Study the drawing (mm; zero at the part's minimum x, y, z) and answer. Coordinates: 2 decimals unless noted, no trailing zeros. Loops run counter-clockwise (first coordinate to the right, second up) from the corner with the lowest first, then second, coordinate; pieces in that order, holes last. Notation, with made-up numbers: (67.5, 84) - (100.5, 84) arc R15 ccw to (100.5, 105) - close; hole circle Ø1 at (77.25, 26). An arc over 180 degrees is marked (long way). Put each result on its own line as item: value.
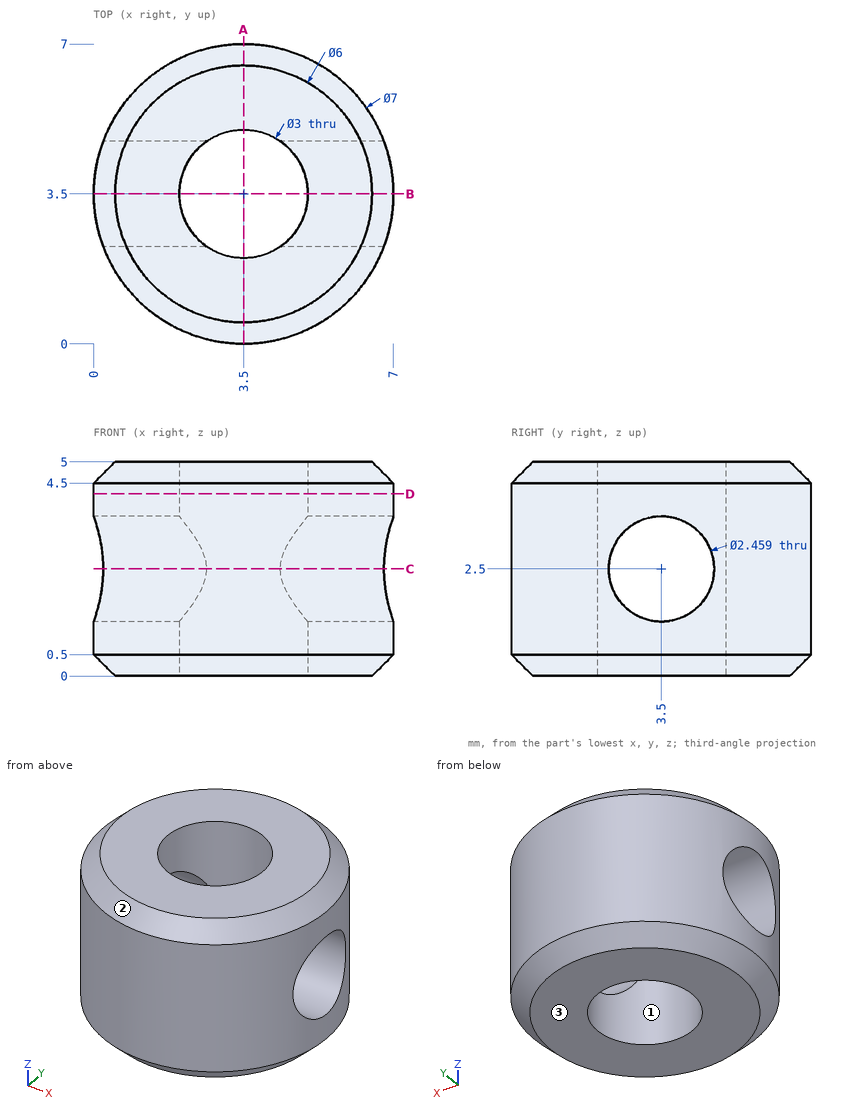
1) For a pull along Y with two mould halves and no side action, classify the marked faces 1, 2 and 3 as pulls with the +Y half, pulls with the -Y half, needs draft (parallel to the pull), parting line crosses it, or undercut.
Found:
face 1: undercut
face 2: parting line crosses it
face 3: needs draft
2) Straight lines are drawn through the part: L1, parallel to Y at x = 3, z = 1.5; L2, parallel to Y at x = 1.25, z = 2.5. For each, find the intervals that lie inside material, in ascending order. Write a range as [from, to].
Found:
L1: y = [0.04, 2.09], [4.91, 6.96]
L2: y = [0.82, 2.27], [4.73, 6.18]
3) The part is cut by section B-B (y = 3.5). Give the vertices of the cut face in (x, z).
Found:
outline: (0, 0.5) - (0.5, 0) - (2, 0) - (2, 1.27) - (0, 1.27) - close; (0, 3.73) - (2, 3.73) - (2, 5) - (0.5, 5) - (0, 4.5) - close; (5, 0) - (6.5, 0) - (7, 0.5) - (7, 1.27) - (5, 1.27) - close; (5, 3.73) - (7, 3.73) - (7, 4.5) - (6.5, 5) - (5, 5) - close
4) Each of these flat-tipped pins is pushed along its axis until it touches: pin 1 (1 mm diameter, centred on x = 6.5, y = 1.5, fed in from +Z); pin 2 (1.8 mm diameter, centred on x = 3.5, y = 3.5, fed in from +Z). Where does it stop, or does it pass through?
Found:
pin 1: stops at z = 4.89
pin 2: passes through
5) The part is cut by section A-A (x = 3.5). Give the vertices of the cut face in (y, z), and give its area (3 significant figures).
Found:
outline: (0, 0.5) - (0.5, 0) - (2, 0) - (2, 5) - (0.5, 5) - (0, 4.5) - close; (5, 0) - (6.5, 0) - (7, 0.5) - (7, 4.5) - (6.5, 5) - (5, 5) - close
area: 19.5 mm^2
6) The part is cut by section D-D (z = 4.25). Give the vertices of the cut face in (x, y), and give its area (3 significant figures).
Found:
outline: circle Ø7 at (3.5, 3.5); hole circle Ø3 at (3.5, 3.5)
area: 31.4 mm^2
7) The part is cut by section C-C (z = 2.5). Give the vertices of the cut face in (x, y).
Found:
outline: (0.22, 2.27) arc R3.5 ccw to (6.78, 2.27) - (4.36, 2.27) arc R1.5 cw to (2.64, 2.27) - close; (0.22, 4.73) - (2.64, 4.73) arc R1.5 cw to (4.36, 4.73) - (6.78, 4.73) arc R3.5 ccw to start
